Can you work these out from the model? Positions are in its coordinate system, mm. A direction names the side the tool comes from. Give positions to 0.01 mm unless a question says otherwise; leave off trailing zeros. Order: outer loops, then holes, each group sorted by start corner. A loop starts at its lowest first (then second) coordinate and runs counter-clockwise, first axis right, second up. Notation, with made-up numbers: (66.5, -28) - (88.5, -28) arc R14 ccw to (88.5, -9) - close; hole circle Ø6 at (56.25, -16). An arc over 180 degrees is marked (long way). Return JSON: item names as keys, results as strings.
```python
from build123d import *

# Parameters (mm, degrees)
F0_W     = 281.3903391361
F0_H     = 488.5678589344
F1_DEPTH = 381
F2_T     = -2.54
F3_W     = 276.3103391361
F3_H     = 15.4284834862
F4_DEPTH = 381


with BuildPart() as f1:
    # F0 (on Front) → F1 (new body)
    with BuildSketch(Plane.XZ):
        with Locations((-45.8520203829, 92.3334807158)):
            Rectangle(F0_W, F0_H)
    extrude(amount=F1_DEPTH)

    # F2
    f2_openings = [f1.faces().sort_by_distance(p)[0] for p in [
        (-45.85202, -381, 92.333481),
    ]]
    offset(amount=F2_T, openings=f2_openings)

    # F3 (on face) → F4 (join)
    with BuildSketch(Plane.XZ.offset(2.54)):
        with Locations((-45.8520203829, 208.1342786551)):
            Rectangle(F3_W, F3_H)
    extrude(amount=F4_DEPTH)


solid = f1.part
```
1. Thinking about a two-plate mould opening in Z: for faces 3 (the face through (-184.007, -189, 274)), 4 (the face through (-48, -383.54, 208)), 5 (the face through (-48, -188, -151.95)), which applies, +Z half, -Z half, draft (parallel to the pull), parting line (faces both ways), or undercut?
Checks:
{"face 3": "undercut", "face 4": "draft", "face 5": "-Z half"}
2. For pin 1 Ø0.8 at (y, z) = (-382, 206.5) entering from +X, with a flat end and sliding along its axis, tell me the tip position at first contact or that it passes through.
Checks:
{"pin 1": "x = 92.3"}
3. If I drill on L1, parallel to Z at x = 72, y = -305.5; L2, parallel to X at y = -217.5, z = -80.5; L3, parallel to Y at x = -42, z = 74, over which ranges is the centre line in solid material (lowest first)? Write a range as [from, to].
Checks:
{"L1": "[-151.95, -149.41], [200.42, 215.85], [334.08, 336.62]", "L2": "[-186.55, -184.01], [92.3, 94.84]", "L3": "[-2.54, 0]"}
4. On a 3-axis mill with a long thin cutter (end or side, diameter ignored), from which of +Z, -Z, +X, -X, +Y, -Y can I reach the whole of each face in a straight line? I mean faces 1 (the face through (-48, -188, 336.617)), 2 (the face through (-48, -2.54, 28)). Say none if no direction works.
Checks:
{"face 1": "+Z, +X, -X, +Y, -Y", "face 2": "-Y"}
5. Suppose I cut it at C-C (z = 223.5). List the corners of the cut face in (x, y) for me.
Checks:
{"outline": "(-186.55, -381) - (-184.01, -381) - (-184.01, -2.54) - (92.3, -2.54) - (92.3, -381) - (94.84, -381) - (94.84, 0) - (-186.55, 0) - close"}
6. Suppose I cut it at A-A (x = -42.5). List the corners of the cut face in (y, z) for me, plus the area to 3 significant figures.
Checks:
{"outline": "(-383.54, 200.42) - (-2.54, 200.42) - (-2.54, -149.41) - (-381, -149.41) - (-381, -151.95) - (0, -151.95) - (0, 336.62) - (-381, 336.62) - (-381, 334.08) - (-2.54, 334.08) - (-2.54, 215.85) - (-383.54, 215.85) - close", "area": "9,040 mm^2"}
7. Suppose I cut it at B-B (y = -112). List the corners of the cut face in (x, z) for me.
Checks:
{"outline": "(-186.55, -151.95) - (94.84, -151.95) - (94.84, 336.62) - (-186.55, 336.62) - close; hole (-184.01, -149.41) - (92.3, -149.41) - (92.3, 200.42) - (-184.01, 200.42) - close; hole (-184.01, 215.85) - (92.3, 215.85) - (92.3, 334.08) - (-184.01, 334.08) - close"}
